The model under review builds one solid part; all positions refer to its coordinate system, in mm. A direction names the side the tool comes from. Round coordinates to 2 decimals unless told otherwise and drop trailing zeros. Write each loop counter-clockwise with the first axis right and the second up, starting at its lowest first coordinate (ties: lowest second). Pieces come first, ordered by that corner, then holes. Notation, with made-up numbers: (62, 43) - (72, 43) arc R15 cw to (72, 71) - close; hole circle Ø5 at (82.25, -13). An arc over 180 degrees is marked (long way). Write each question's results on one line, items separated by ' | '.
```python
from build123d import *

# Parameters (mm, degrees)
BOX003_W     = 10
BOX003_H     = 10
BOX003_DEPTH = 8
BOX002_W     = 8
BOX002_H     = 8
BOX002_DEPTH = 20
BOX_W        = 16
BOX_H        = 16
BOX_DEPTH    = 10


with BuildPart() as cube001:
    # Box003 → Box003 (new body)
    with BuildSketch(Plane(origin=(-5, -5, 0), x_dir=(1, 0, 0), z_dir=(0, 0, 1))):
        with Locations((5, 5)):
            Rectangle(BOX003_W, BOX003_H)
    extrude(amount=BOX003_DEPTH)


with BuildPart() as body:
    # Box002 → Box002 (join)
    with BuildSketch(Plane(origin=(-4, -4, 0), x_dir=(1, 0, 0), z_dir=(0, 0, 1))):
        with Locations((4, 4)):
            Rectangle(BOX002_W, BOX002_H)
    extrude(amount=BOX002_DEPTH)

    # Sphere → Sphere (revolve, cut)
    with BuildSketch(Plane(origin=(0, 0, 20), x_dir=(1, 0, 0), z_dir=(0, -1, 0))):
        with BuildLine():
            ThreePointArc((0, -2), (2, 0), (0, 2))
            Line((0, 2), (0, -2))
        make_face()
    revolve(axis=Axis((0, 0, 20), (0, 0, 1)), mode=Mode.SUBTRACT)


with BuildPart() as cut:
    # Box → Box (new body)
    with BuildSketch(Plane(origin=(-8, -8, 0), x_dir=(1, 0, 0), z_dir=(0, 0, 1))):
        with Locations((8, 8)):
            Rectangle(BOX_W, BOX_H)
    extrude(amount=BOX_DEPTH)

    # Fusion: union Body
    add(body.part)

    # Cut: cut Cube001
    add(cube001.part, mode=Mode.SUBTRACT)


solid = cut.part
```
Q1. For probe 1 along X at (y, z) = (0, 2.75); probe 2 along Y at (x, z) = (-0.75, 17), list the stretches that pass through material, from the lowest coordinate up.
Evaluation:
probe 1: x = -8 to -5, 5 to 8 | probe 2: y = -4 to 4
Q2. We need section D-D (z = 14.25). State the section outline as (x, y) points.
Evaluation:
outline: (-4, -4) - (4, -4) - (4, 4) - (-4, 4) - close
Q3. We need section B-B (x = -4.5). State the section outline as (y, z) points, plus the area to 3 significant figures.
Evaluation:
outline: (-8, 0) - (-5, 0) - (-5, 8) - (5, 8) - (5, 0) - (8, 0) - (8, 10) - (-8, 10) - close | area: 80.0 mm^2
Q4. The part is to be moulded in two halves that separate along X. For faces 1 (the flat face through (0, -4, 15)), 2 (the flat face through (0, -5, 4)), 3 (the flat face through (4, 0, 15)), say which applies: released by +X, released by -X, zero draft, split by the parting line, or undercut.
Evaluation:
face 1: zero draft | face 2: undercut | face 3: released by +X
Q5. We need section C-C (y = -0.25). State the section outline as (x, z) points, plus the area to 3 significant figures.
Evaluation:
outline: (-8, 0) - (-5, 0) - (-5, 8) - (5, 8) - (5, 0) - (8, 0) - (8, 10) - (4, 10) - (4, 20) - (1.98, 20) arc R1.98 cw to (-1.98, 20) - (-4, 20) - (-4, 10) - (-8, 10) - close | area: 154 mm^2
Q6. Tool access review of faces 4 (the flat face through (0, 5, 4)), 5 (the flat face through (0, 5, 10)), 6 (the flat face through (-4, 0, 15)), 7 (the flat face through (0, 4, 15)), 8 (the flat face through (-2, 1, 20)): name each direction out of +Z, -Z, +X, -X, +Y, -Y from which nothing blocks a thin tool from reaching the whole face with its end or side.
Evaluation:
face 4: -Z | face 5: +Z | face 6: +Z, -X, +Y, -Y | face 7: +Z, +X, -X, +Y | face 8: +Z, +X, -X, +Y, -Y
Q7. We need section A-A (z = 7.5). State the section outline as (x, y) points, plus the area to 3 significant figures.
Evaluation:
outline: (-8, -8) - (8, -8) - (8, 8) - (-8, 8) - close; hole (-5, -5) - (5, -5) - (5, 5) - (-5, 5) - close | area: 156 mm^2
Q8. Insertion check: P1, Ø1, axis at x = 1, y = -2, coming from the -Z side; P2, Ø6.5, axis at x = 1.5, z = 16, coming from the +Y side; P3, Ø2.5, axis at x = -1, z = 12.5, coming from the -Y side. Each pin has a flat end and moves straight along its axis. Give the tip position at first contact, or say it passes through.
Evaluation:
P1: stops at z = 8 | P2: stops at y = 4 | P3: stops at y = -4
